Part print with two shaded views. Sizes in mm from the minimum x, y, z corner. A direction names the side the tool comes from. Round coordinates to 2 decimals unless told otherwise and drop trailing zeros. Order: outer loops, then holes, each group sorted by start corner. A loop starts at its lowest first (then second) coordinate and runs counter-clockwise, first axis right, second up. Notation, with made-up numbers: M 77.25,24.5 L 106.25,24.5 A16 ccw 106.25,42.5 Z; hole C 59,-20 d4. An arc over 180 degrees is marked long. Answer as a JSON object with one key per item and string values.
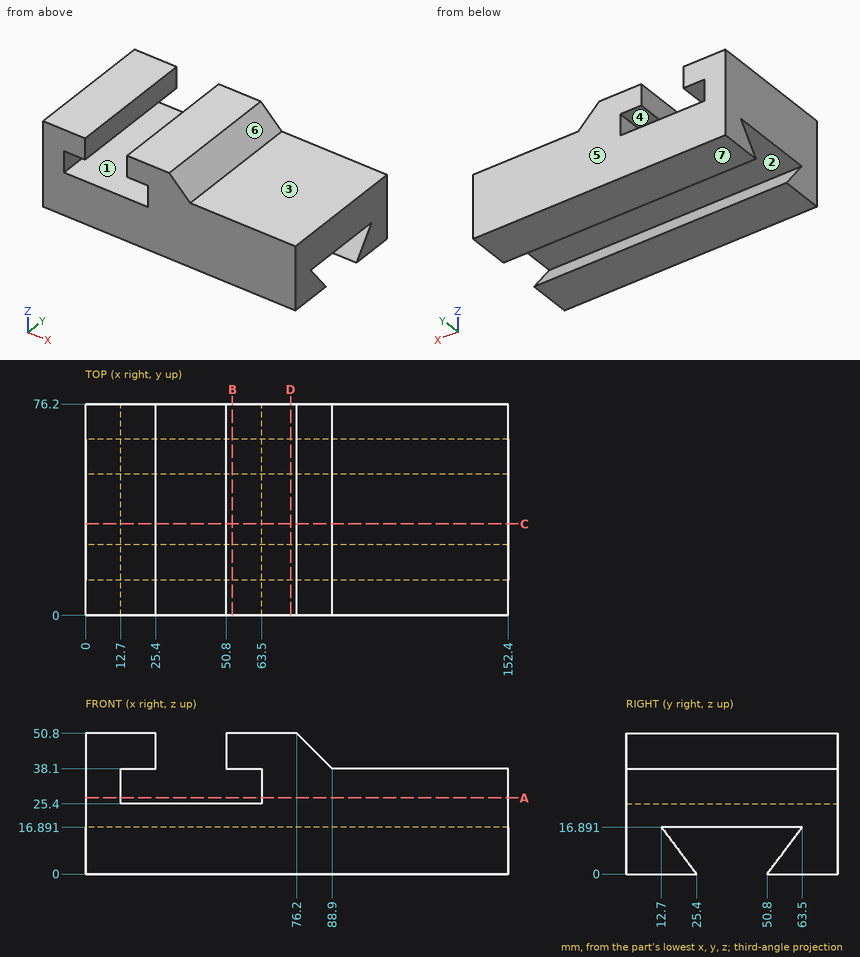
Item 1: Saw through at A-A on z = 27.5. List the corners of the cut face in (x, y), and give its area (3 significant figures).
Worked answers:
{"outline": "M 0,0 L 12.7,0 L 12.7,76.2 L 0,76.2 Z; M 63.5,0 L 152.4,0 L 152.4,76.2 L 63.5,76.2 Z", "area": "7,740 mm2"}
Item 2: Wall check: line 1 along X through (y, z) = (20, 26); line 2 along Z through (x, y) = (127.5, 50); line 3 along Z through (x, y) = (52, 68). Give the ranges that are in metal, low to high. Write a range as [from, to].
Worked answers:
{"line 1": "x = [0, 12.7], [63.5, 152.4]", "line 2": "z = [16.89, 38.1]", "line 3": "z = [0, 25.4], [38.1, 50.8]"}
Item 3: Saw through at D-D on x = 74. List the corners of the cut face in (y, z), and give its area (3 significant figures).
Worked answers:
{"outline": "M 0,0 L 25.4,0 L 12.7,16.89 L 63.5,16.89 L 50.8,0 L 76.2,0 L 76.2,50.8 L 0,50.8 Z", "area": "3,230 mm2"}
Item 4: Two-plate mould, pull along Z, no slides. Class the marked faces 4, 5, 6 and 7: released by +Z, released by -Z, zero draft, split by the parting line, or undercut.
Worked answers:
{"face 4": "undercut", "face 5": "zero draft", "face 6": "released by +Z", "face 7": "released by -Z"}
Item 5: Saw through at C-C on y = 33. List the corners of the cut face in (x, z).
Worked answers:
{"outline": "M 0,16.89 L 152.4,16.89 L 152.4,38.1 L 88.9,38.1 L 76.2,50.8 L 50.8,50.8 L 50.8,38.1 L 63.5,38.1 L 63.5,25.4 L 12.7,25.4 L 12.7,38.1 L 25.4,38.1 L 25.4,50.8 L 0,50.8 Z"}
Item 6: 3-axis set-ups, long thin cutter, end or side, ignore diameter. For the marked faces 1, 2 and 3: which of +Z, -Z, +X, -X, +Y, -Y reach the whole face in a straight line?
Worked answers:
{"face 1": "+Y, -Y", "face 2": "+X, -X", "face 3": "+Z, +X, +Y, -Y"}
Item 7: Drop flat-ended pins along their axis: pin 1 Ø6.5 at (x, y) = (59, 42.5) entering from -Z; pin 2 Ø12 at (x, y) = (78, 17) entering from +Z; pin 3 Ø6.5 at (y, z) = (27, 42) entering from +X; pin 4 Ø10 at (x, z) = (34, 43) entering from -Y. Give the stop position or say it passes through.
Worked answers:
{"pin 1": "stops at z = 16.89", "pin 2": "stops at z = 50.8", "pin 3": "stops at x = 88.25", "pin 4": "passes through"}
Item 8: Saw through at B-B on x = 53. List the corners of the cut face in (y, z), and give its area (3 significant figures).
Worked answers:
{"outline": "M 0,0 L 25.4,0 L 12.7,16.89 L 63.5,16.89 L 50.8,0 L 76.2,0 L 76.2,25.4 L 0,25.4 Z; M 0,38.1 L 76.2,38.1 L 76.2,50.8 L 0,50.8 Z", "area": "2,260 mm2"}
